Here's how the part is built. I have some questions about the finished solid (model axes, mm). Round coordinates to 2 decimals unless told otherwise and drop trailing zeros. Loops run counter-clockwise (first coordinate to the right, second up) from the corner with the lowest first, then second, coordinate; pieces in that order, holes last. Notation, with made-up numbers: (36.25, 88.5) -> (46.25, 88.5) arc R25 cw to (46.25, 108.5) -> close; hole circle Ø3 at (30, 21). An arc over 180 degrees is marked (long way). Use one line per item in the form item = value. Start each with the question number.
Item 1: If I drill on L1, parallel to Z at x = -125, y = 1.65; L2, parallel to X at y = 1.7, z = -97.5; L3, parallel to Y at x = 26.5, z = 89, over which ranges is the centre line in solid material (lowest first)? Write a range as [from, to].
Item 2: If we section it at A-A (z = -30): Write out the boundary of the cut face in (x, y), then the cut area to 3 significant figures.
Item 3: I'm going to push a flat-ended pin straight in: pin 1 Ø4 at (x, z) = (32.5, -51) entering from +Y. Where does the tip first touch, or does it pass through?
Item 4: Thinking about a two-plate mould opening in Z: for faces 1 (the face through (-2, 1.5, -2)), 2 (the face through (13, 2, -118)), which applies, released by +Z, released by -Z, zero draft, split by the parting line, or undercut?
Item 5: If we section it at B-B (x = 36.5): Write out the boundary of the cut face in (y, z), then the cut area to 3 significant figures.
Autodesk Inventor part; units mm, degrees
ref_plane "YZ Plane" through (0, 0, 0) normal (1, 0, 0) x (0, 1, 0)
ref_plane "XZ Plane" through (0, 0, 0) normal (0, 1, 0) x (-1, 0, 0)
ref_plane "XY Plane" through (0, 0, 0) normal (0, 0, 1) x (1, 0, 0)
sketch "Szkic1" plane through (0, 0, 0) normal (0, 1, 0) x (-1, 0, 0)
  line L0 (-161, -123.5) -> (161, -123.5)
  line L1 (161, -123.5) -> (161, 123.5)
  line L2 (161, 123.5) -> (-161, 123.5)
  line L3 (-161, 123.5) -> (-161, -123.5)
  line L4 (-161, -123.5) -> (161, 123.5) construction
  line L5 (161, -123.5) -> (-161, 123.5) construction
  point P0 (0, 0)
  dimension "d0" = 322
  dimension "d1" = 247
extrude "Wyciągnięcie proste1" add sketch "Szkic1" along normal blind 2
sketch "Szkic2" plane through (0, 2, 0) normal (0, 1, 0) x (1, 0, 0)
  line L0 (161, 123.5) -> (-161, 123.5)
  line L1 (-161, 123.5) -> (-161, -123.5)
  line L2 (-161, -123.5) -> (161, -123.5)
  line L3 (161, -123.5) -> (161, 123.5)
  line L4 (152, 114) -> (-152, 114)
  line L5 (-152, 114) -> (-152, -114)
  line L6 (-152, -114) -> (152, -114)
  line L7 (152, -114) -> (152, 114)
  line L8 (152, 114) -> (-152, -114) construction
  line L9 (-152, 114) -> (152, -114) construction
  point P0 (0, 0)
  dimension "d11" = 9
  dimension "d12" = 9
  dimension "d13" = 9.5
  dimension "d14" = 9.5
extrude "Wyciągnięcie proste3" cut sketch "Szkic2" against normal blind 0.5 contours L7 L6 L5 L4
equation "\"d14\" = d13"
properties part number "resistive_panel_12.1" material "Szkło"
Values found:
q1.L1 = [-123.5, -114], [114, 123.5]
q1.L2 = [-161, -152], [152, 161]
q1.L3 = [0, 1.5]
q2.outline = (-161, 0) -> (161, 0) -> (161, 2) -> (152, 2) -> (152, 1.5) -> (-152, 1.5) -> (-152, 2) -> (-161, 2) -> close
q2.area = 492 mm2
q3.pin_1 = 1.5
q4.face_1 = undercut
q4.face_2 = zero draft
q5.outline = (0, -123.5) -> (2, -123.5) -> (2, -114) -> (1.5, -114) -> (1.5, 114) -> (2, 114) -> (2, 123.5) -> (0, 123.5) -> close
q5.area = 380 mm2
